Here's how the part is built. I have some questions about the finished solid (model axes, mm). Face numbers are marked on the shaded views. A direction names the side the tool comes from. Coordinates: 2 decimals unless noted, no trailing zeros. Loops run counter-clockwise (first coordinate to the right, second up) from the corner with the lowest first, then second, coordinate; pieces in that order, holes last.
from build123d import *

# Parameters (mm, degrees)
BOSS_EXTRUDE1_DEPTH = 1
SKETCH2_R           = 3.15
BOSS_EXTRUDE2_DEPTH = 6.7
FILLET1_R           = 0.5


with BuildPart() as part:
    # Sketch1 → Boss-Extrude1 (new body)
    with BuildSketch(Plane(origin=(0, 0, 0), x_dir=(1, 0, 0), z_dir=(0, 1, 0))):
        Polygon((-1.562548269, 3.3), (-3.3, 1.562548269), (-3.3, -3.3), (3.3, -3.3), (3.3, 1.562548269), (1.562548269, 3.3), align=None)
    extrude(amount=BOSS_EXTRUDE1_DEPTH)

    # Sketch2 → Boss-Extrude2 (add)
    with BuildSketch(Plane(origin=(0, 1, 0), x_dir=(-1, 0, 0), z_dir=(0, 1, 0))):
        Circle(SKETCH2_R)
    extrude(amount=BOSS_EXTRUDE2_DEPTH)

    # Fillet1
    fillet1_edges = [part.edges().sort_by_distance(p)[0] for p in [
        (3.15, 7.7, 0),
    ]]
    fillet(fillet1_edges, radius=FILLET1_R)


solid = part.part
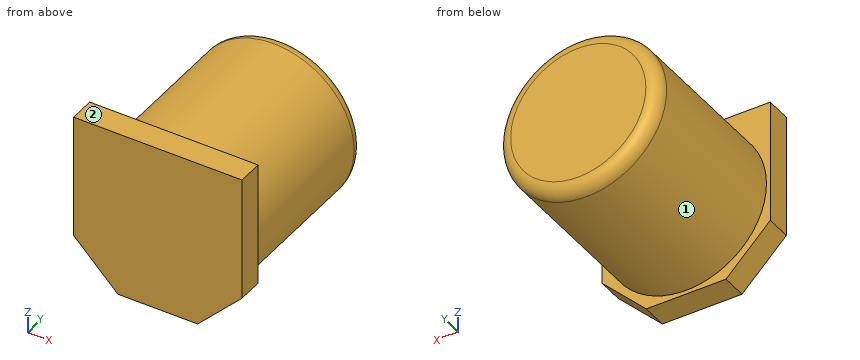
Q1. For the marked faces 1 and 2, which set-ups out of +Z, -Z, +X, -X, +Y, -Y let a thin tool reach every point of the face, with its end or its side?
Q2. Please list where these lines run through material, in increasing order: probe 1 along Y at (x, z) = (3, -1.5); probe 2 along Y at (x, z) = (-1.5, -2.25); probe 3 along Z at (x, y) = (2.5, 6.5).
Q3. Suppose I cut it at C-C on y = 2. Write out the boundary of the cut face in (x, z).
Q4. Will this pin go through, and if not, where does the flat tip stop? P1, Ø2, axis at x = 0.5, y = 5.5, coming from the -Z side.
Q5. Suppose I cut it at A-A on z = 0. Write out the boundary of the cut face in (x, y).
Q6. Suppose I cut it at B-B on x = 0. Write out the boundary of the cut face in (y, z).
Check values:
1. face 1: +Y
1. face 2: +Z, +X, -X, +Y, -Y
2. probe 1: y = 0 to 1
2. probe 2: y = 0 to 7.7
2. probe 3: z = -1.92 to 1.92
3. outline: circle Ø6.3 at (0, 0)
4. P1: stops at z = -3.15
5. outline: (-3.3, 0) - (3.3, 0) - (3.3, 1) - (3.15, 1) - (3.15, 7.2) arc R0.5 ccw to (2.65, 7.7) - (-2.65, 7.7) arc R0.5 ccw to (-3.15, 7.2) - (-3.15, 1) - (-3.3, 1) - close
6. outline: (0, -3.3) - (1, -3.3) - (1, -3.15) - (7.2, -3.15) arc R0.5 ccw to (7.7, -2.65) - (7.7, 2.65) arc R0.5 ccw to (7.2, 3.15) - (1, 3.15) - (1, 3.3) - (0, 3.3) - close
